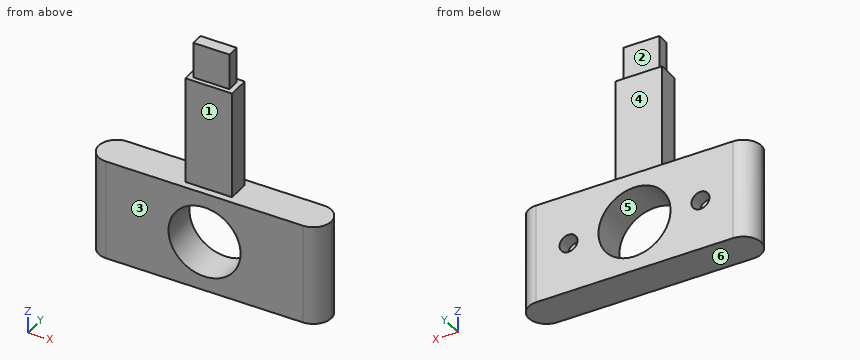
```python
from build123d import *

# Parameters (mm, degrees)
BOSS_EXTRUDE1_DEPTH = 35.56
SKETCH2_W           = 16.51
SKETCH2_H           = 38.1
BOSS_EXTRUDE2_DEPTH = 12.7
SKETCH3_W           = 38.1
SKETCH3_H           = 2.54
CUT_EXTRUDE1_DEPTH  = 50.276
SKETCH4_W           = 12.7
SKETCH4_H           = 4.318
BOSS_EXTRUDE3_DEPTH = 12.7
SKETCH5_R           = 12.7
CUT_EXTRUDE2_DEPTH  = 13.7
SKETCH6_R           = 3.175
CUT_EXTRUDE3_DEPTH  = 5.08


with BuildPart() as part:
    # Sketch1 → Boss-Extrude1 (new body)
    with BuildSketch(Plane.XY):
        with BuildLine():
            ThreePointArc((0, 6.35), (1.859871939, 1.859871939), (6.35, 0))
            Line((6.35, 0), (75.692, 0))
            ThreePointArc((75.692, 0), (80.182128061, 1.859871939), (82.042, 6.35))
            ThreePointArc((82.042, 6.35), (80.182128061, 10.840128061), (75.692, 12.7))
            Line((75.692, 12.7), (6.35, 12.7))
            ThreePointArc((6.35, 12.7), (1.859871939, 10.840128061), (0, 6.35))
        make_face()
    extrude(amount=BOSS_EXTRUDE1_DEPTH)

    # Sketch2 → Boss-Extrude2 (add)
    with BuildSketch(Plane(origin=(0, 12.7, 0), x_dir=(1, 0, 0), z_dir=(0, 1, 0))):
        with Locations((41.021, -54.61)):
            Rectangle(SKETCH2_W, SKETCH2_H)
    extrude(amount=-BOSS_EXTRUDE2_DEPTH)

    # Sketch3 → Cut-Extrude1 (cut, through all)
    with BuildSketch(Plane.ZY.offset(-32.766)):
        with Locations((54.61, 11.43)):
            Rectangle(SKETCH3_W, SKETCH3_H)
        with Locations((54.61, 1.27)):
            Rectangle(SKETCH3_W, SKETCH3_H)
    extrude(amount=-CUT_EXTRUDE1_DEPTH, mode=Mode.SUBTRACT)

    # Sketch4 → Boss-Extrude3 (add)
    with BuildSketch(Plane.XY.offset(73.66)):
        with Locations((41.021, 6.35)):
            Rectangle(SKETCH4_W, SKETCH4_H)
    extrude(amount=BOSS_EXTRUDE3_DEPTH)

    # Sketch5 → Cut-Extrude2 (cut, through all)
    with BuildSketch(Plane(origin=(0, 12.7, 0), x_dir=(1, 0, 0), z_dir=(0, 1, 0))):
        with Locations((41.021, -17.78)):
            Circle(SKETCH5_R)
    extrude(amount=-CUT_EXTRUDE2_DEPTH, mode=Mode.SUBTRACT)

    # Sketch6 → Cut-Extrude3 (cut)
    with BuildSketch(Plane(origin=(0, 12.7, 0), x_dir=(1, 0, 0), z_dir=(0, 1, 0))):
        with Locations((64.262, -17.78)):
            Circle(SKETCH6_R)
        with Locations((17.78, -17.78)):
            Circle(SKETCH6_R)
    extrude(amount=-CUT_EXTRUDE3_DEPTH, mode=Mode.SUBTRACT)


solid = part.part
```
Check sheet for the modelled part. Datum: model origin and axes. Units: mm. Face numbers are marked on the shaded views. A direction names the side the tool comes from. Give positions to 0.01 mm unless a question says otherwise; leave off trailing zeros. Write each loop counter-clockwise with the first axis right and the second up, starting at its lowest first coordinate (ties: lowest second). Pieces come first, ordered by that corner, then holes. Notation, with made-up numbers: (72.25, 37) - (84.25, 37) arc R4 ccw to (84.25, 44) - close; hole circle Ø11 at (52, 47.5). An arc over 180 degrees is marked (long way). Answer as a JSON object with one key per item and string values. Group by question number.
1) Thickness scan on probe 1 along X at (y, z) = (8.7, 17.78) (3 decimals); probe 2 along X at (y, z) = (9.2, 17.78) (1 decimal); probe 3 along X at (y, z) = (3, 52). Record the ranges inside material, lowest first. Write a range as from..to.
2) Sectioned sample at B-B (x = 38.5). Record the cut outline in (y, z), then the cut area to 3 significant figures.
3) Sectioned sample at A-A (z = 17.78). Record the cut outline in (x, y) (3 decimals), then the cut area to 3 significant figures.
4) Sectioned sample at C-C (x = 17.78). Record the cut outline in (y, z) (3 decimals).
5) Access from +Z, -Z, +X, -X, +Y, -Y to the whole of each face (thin tool, end or side, straight path). Record for the marked faces 1, 2 and 3.
6) Depth check by flat-ended pin: P1, Ø6, axis at y = 9, z = 67, coming from the -X side; P2, Ø10, axis at x = 42.5, z = 82, coming from the -Y side; P3, Ø1.3, axis at y = 6, z = 77, coming from the +X side; P4, Ø20.5, axis at x = 41.021, z = 17.78, coming from the +Y side. Enter the tip coordinate at first touch or a pass-through.
7) Sectioned sample at D-D (y = 1). Record the cut outline in (x, z), then the cut area to 3 significant figures.
8) Release check for a two-part mould opening along Z. For the marked faces 4, 5 and 6 record: pulls with the +Z half, pulls with the -Z half, needs draft (parallel to the pull), parting line crosses it, or undercut.
Geometry results:
{
 "1": {"probe 1": "x = 0.451..14.605, 20.955..28.321, 53.721..61.087, 67.437..81.591", "probe 2": "x = 0.7..14.6, 21..28.3, 53.7..61.1, 67.4..81.4", "probe 3": "x = 32.77..49.28"},
 "2": {"outline": "(0, 0) - (12.7, 0) - (12.7, 5.33) - (0, 5.33) - close; (0, 30.23) - (12.7, 30.23) - (12.7, 35.56) - (10.16, 35.56) - (10.16, 73.66) - (8.51, 73.66) - (8.51, 86.36) - (4.19, 86.36) - (4.19, 73.66) - (2.54, 73.66) - (2.54, 35.56) - (0, 35.56) - close", "area": "481 mm^2"},
 "3": {"outline": "(6.35, 0) - (28.321, 0) - (28.321, 12.7) - (20.955, 12.7) - (20.955, 7.62) - (14.605, 7.62) - (14.605, 12.7) - (6.35, 12.7) arc R6.35 ccw to start; (53.721, 0) - (75.692, 0) arc R6.35 ccw to (75.692, 12.7) - (67.437, 12.7) - (67.437, 7.62) - (61.087, 7.62) - (61.087, 12.7) - (53.721, 12.7) - close", "area": "620 mm^2"},
 "4": {"outline": "(0, 0) - (12.7, 0) - (12.7, 14.605) - (7.62, 14.605) - (7.62, 20.955) - (12.7, 20.955) - (12.7, 35.56) - (0, 35.56) - close"},
 "5": {"face 1": "+Z, +X, -X, -Y", "face 2": "+Z, +X, -X, +Y", "face 3": "+Z, -Z, +X, -X, -Y"},
 "6": {"P1": "stops at x = 32.77", "P2": "stops at y = 4.19", "P3": "stops at x = 47.37", "P4": "passes through"},
 "7": {"outline": "(2.93, 0) - (79.11, 0) - (79.11, 35.56) - (2.93, 35.56) - close; hole circle Ø25.4 at (41.02, 17.78)", "area": "2,200 mm^2"},
 "8": {"face 4": "needs draft", "face 5": "undercut", "face 6": "pulls with the -Z half"}
}
